Job drawing, mm, ordinate dimensions from the low corner. One solid piece. Round coordinates to 2 decimals unless told otherwise and drop trailing zeros. Write each loop counter-clockwise with the first axis right and the second up, starting at its lowest first coordinate (ties: lowest second). Pieces come first, ordered by that corner, then holes.
1) Saw through at D-D on y = 1.55. Count the separate pieces of the cut face and the enclosed holes in it, and give its area (3 significant figures).
2) Flat gauge pins, fed straight in: pin 1 (0.9 mm diameter, centred on x = 173, y = 1, fed in from -Z); pin 2 (0.9 mm diameter, centred on y = 2, z = 39.5, fed in from -X); pin 3 (10 mm diameter, centred on x = 47, z = 32, fed in from -Y). Where does each tip first touch, or does it go through?
3) Saw through at C-C on x = 73. Write the cut outline in (y, z).
4) Saw through at B-B on z = 15.5. Write the cut outline in (x, y) (1 decimal).
5) Saw through at A-A on x = 127.5. Write the cut outline in (y, z).
6) Drill centre lines: L1, parallel to Z at x = 119, y = 2.95; L2, parallel to Z at x = 83.5, y = 0.5; L3, parallel to X at y = 1.4, z = 28 (1 decimal). Where is each one in solid material? Low to high.
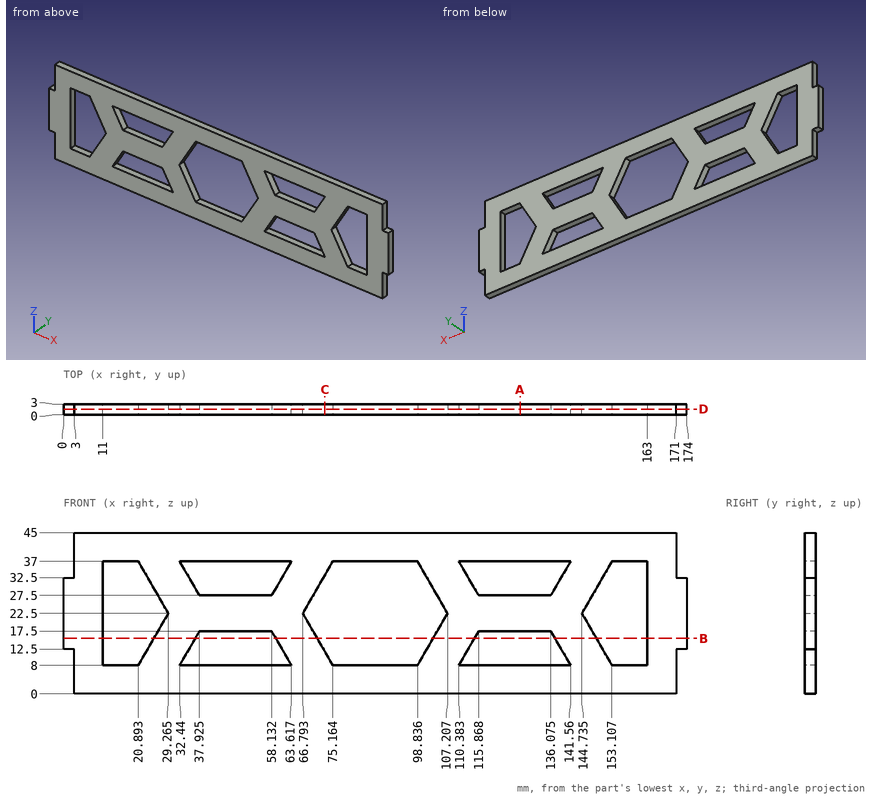
Completed:
1. separate pieces: 1
1. enclosed holes: 7
1. area: 4,960 mm2
2. pin 1: stops at z = 12.5
2. pin 2: stops at x = 3
2. pin 3: stops at y = 0
3. outline: (0, 0) - (3, 0) - (3, 11.75) - (0, 11.75) - close; (0, 33.25) - (3, 33.25) - (3, 45) - (0, 45) - close
4. outline: (0, 0) - (11, 0) - (11, 3) - (0, 3) - close; (25.2, 0) - (36.8, 0) - (36.8, 3) - (25.2, 3) - close; (59.3, 0) - (70.8, 0) - (70.8, 3) - (59.3, 3) - close; (103.2, 0) - (114.7, 0) - (114.7, 3) - (103.2, 3) - close; (137.2, 0) - (148.8, 0) - (148.8, 3) - (137.2, 3) - close; (163, 0) - (174, 0) - (174, 3) - (163, 3) - close
5. outline: (0, 0) - (3, 0) - (3, 8) - (0, 8) - close; (0, 17.5) - (3, 17.5) - (3, 27.5) - (0, 27.5) - close; (0, 37) - (3, 37) - (3, 45) - (0, 45) - close
6. L1: z = 0 to 8, 17.5 to 27.5, 37 to 45
6. L2: z = 0 to 8, 37 to 45
6. L3: x = 0 to 11, 26.1 to 37.6, 58.4 to 70, 104 to 115.6, 136.4 to 147.9, 163 to 174
